The model under review builds one solid part; all positions refer to its coordinate system, in mm. A direction names the side the tool comes from. Round coordinates to 2 decimals unless told otherwise and drop trailing zeros. Write each loop counter-clockwise with the first axis right and the second up, starting at its lowest first coordinate (ties: lowest second). Pieces come first, ordered by that corner, then holes. Notation, with made-up numbers: M 27.25,44 L 56.25,44 A23 cw 56.25,76 Z; hole C 15,1 d2. An arc over 180 degrees is marked long. One line per item, written item: value. Start each with the question number.
1) Tool access review of faces 1 (the face through (0, 2, 23)), 2 (the face through (-7.123, -11.172, 42.986)), 3 (the face through (-6, 3, 42)): name each direction out of +Z, -Z, +X, -X, +Y, -Y from which nothing blocks a thin tool from reaching the whole face with its end or side.
2) Take a section at A-A, the plane x = 0. Write out the cut boundary in (y, z).
3) Mouldability with a two-part tool opening along Y and no side actions: class faces 4 (the face through (6, 0, 21)), 5 (the face through (0, 0, 3)), 6 (the face through (0, 0, 0)) as +Y half, -Y half, draft (parallel to the pull), parting line (faces both ways), or undercut.
4) Take a section at C-C, the plane z = 37.5. Write out the cut boundary in (x, y), and give its area (3 significant figures).
5) Wall thickness on probe 1 along X at (y, z) = (0, 13.5); probe 2 along X at (y, z) = (-0.75, 8): over which ranges is each line inside the solid? List them lowest first.
6) For P1, Ø5, axis at x = 2.5, y = 8.5, coming from the -Z side; P2, Ø1.5, axis at x = 5.5, y = -2.5, coming from the -Z side; P3, Ø2, axis at x = 6.5, z = 40, coming from the -Y side; P4, Ø2, axis at x = -0.5, y = -4.5, coming from the +Z side, all flat-tipped, find the tip position at first contact; note any pin that passes through.
from build123d import *

# Parameters (mm, degrees)
F2_R = 1


with BuildPart() as f1:
    # F0 (on Front) → F1 (revolve)
    with BuildSketch(Plane.XZ):
        Polygon((-6, 0), (0, 0), (0, 3), (-2, 3), (-2, 42), (-5, 45), (-13.25, 45), (-13.25, 42), (-6, 42), align=None)
    revolve(axis=Axis((0, 0, 1.5), (0, 0, 1)))

    # F2
    f2_edges = [f1.edges().sort_by_distance(p)[0] for p in [
        (6, 0, 0),
        (13.25, 0, 45),
    ]]
    fillet(f2_edges, radius=F2_R)


solid = f1.part
Checked values:
1. face 1: +Z
1. face 2: +Z, -Z
1. face 3: -Z
2. outline: M -13.25,42 L -6,42 L -6,1 A1 ccw -5,0 L 5,0 A1 ccw 6,1 L 6,42 L 13.25,42 L 13.25,44 A1 ccw 12.25,45 L 5,45 L 2,42 L 2,3 L -2,3 L -2,42 L -5,45 L -12.25,45 A1 ccw -13.25,44 Z
3. face 4: parting line
3. face 5: undercut
3. face 6: draft
4. outline: C 0,0 d12; hole C 0,0 d4
4. area: 101 mm2
5. probe 1: x = -6 to -2, 2 to 6
5. probe 2: x = -5.95 to -1.85, 1.85 to 5.95
6. P1: stops at z = 42
6. P2: stops at z = 0.04
6. P3: stops at y = -2.4
6. P4: stops at z = 45
